Can you work these out from the drawing? Everything is in mm from the part's minimum corner. A direction names the side the tool comes from. Give positions to 0.01 mm unless a question says otherwise; leave off trailing zeros. Order: outer loops, then holes, each group sorted by start corner. A loop starts at its lowest first (then second) coordinate and runs counter-clockwise, first axis right, second up. Notation, with made-up numbers: M 55.5,86.25 L 95.5,86.25 A17 cw 95.5,102.25 Z; hole C 46.25,77 d3. An arc over 180 degrees is marked long. Answer in a Markdown table with one row per item. Add a question column.
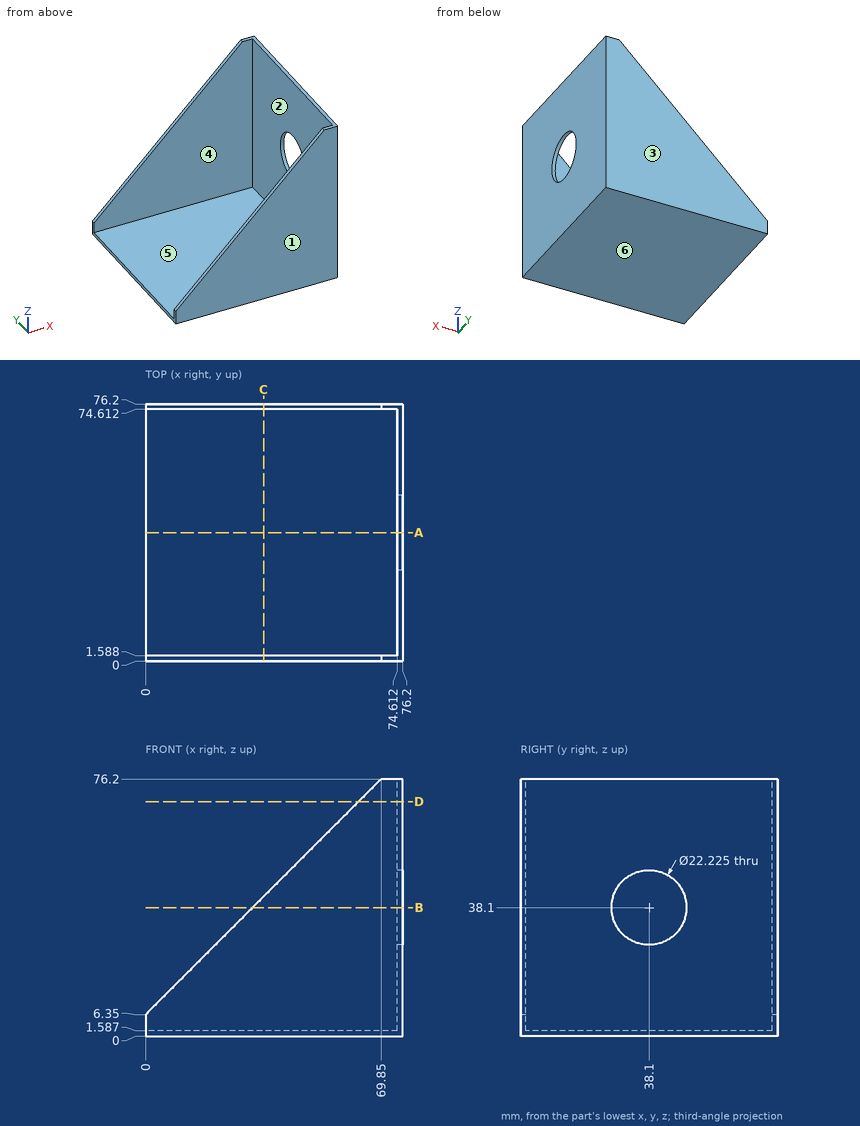
1. Thinking about a two-plate mould opening in Y: for the marked faces 3, 4, 5 and 6, which applies, pulls with the +Y half, pulls with the -Y half, needs draft (parallel to the pull), parting line crosses it, or undercut?
2. Suppose I cut it at D-D on z = 69.5. List the corners of the cut face in (x, y) for me.
3. Will this pin go through, and if not, where does the flat tip stop? P1, Ø22, axis at x = 21.5, y = 31.5, coming from the +Z side.
4. Suppose I cut it at A-A on y = 38.1. List the corners of the cut face in (x, z) for me.
5. If I drill on line 1 along Y through (x, z) = (75, 38); line 2 along Y through (x, z) = (7, 8), over which ranges is the centre line in solid material (lowest first)? Write a range as [from, to].
6. Suppose I cut it at C-C on x = 35. List the corners of the cut face in (y, z) for me.
7. Suppose I cut it at B-B on z = 38.1. List the corners of the cut face in (x, y) for me.
8. For the marked faces 1 and 2, which set-ups out of +Z, -Z, +X, -X, +Y, -Y let a thin tool reach every point of the face, with its end or its side?
Findings below:
| question | item | result |
|---|---|---|
| 1 | face 3 | pulls with the +Y half |
| 1 | face 4 | undercut |
| 1 | face 5 | undercut |
| 1 | face 6 | needs draft |
| 2 | outline | M 63.15,0 L 76.2,0 L 76.2,76.2 L 63.15,76.2 L 63.15,74.61 L 74.61,74.61 L 74.61,1.59 L 63.15,1.59 Z |
| 3 | P1 | z = 1.59 |
| 4 | outline | M 0,0 L 76.2,0 L 76.2,26.99 L 74.61,26.99 L 74.61,1.59 L 0,1.59 Z; M 74.61,49.21 L 76.2,49.21 L 76.2,76.2 L 74.61,76.2 Z |
| 5 | line 1 | [0, 26.99], [49.21, 76.2] |
| 5 | line 2 | [0, 1.59], [74.61, 76.2] |
| 6 | outline | M 0,0 L 76.2,0 L 76.2,41.35 L 74.61,41.35 L 74.61,1.59 L 1.59,1.59 L 1.59,41.35 L 0,41.35 Z |
| 7 | outline | M 31.75,0 L 76.2,0 L 76.2,26.99 L 74.61,26.99 L 74.61,1.59 L 31.75,1.59 Z; M 31.75,74.61 L 74.61,74.61 L 74.61,49.21 L 76.2,49.21 L 76.2,76.2 L 31.75,76.2 Z |
| 8 | face 1 | +Z, -Z, +X, -X, -Y |
| 8 | face 2 | +Z, -X |
